Could you check a few things on this model? Use its own coordinates, in mm. A direction names the side the tool comes from. Coordinates: 2 decimals unless noted, no trailing zeros. Write each loop counter-clockwise with the first axis right and the second up, starting at its lowest first coordinate (ties: lowest second). Pieces come first, ordered by that corner, then holes.
Item 1: I want a section at A-A on z = -30. Please give me the cut outline in (x, y), then the cut area to 3 significant figures.
Item 2: I want a section at C-C on y = 13.5. Please give me the cut outline in (x, z), then the cut area to 3 significant figures.
Item 3: Which directions (+Z, -Z, +X, -X, +Y, -Y) give clear straight access to the entire face, cutting with the end or side of a thin tool? Please do faces 1 (the flat face through (16.35, 17, -27)), 2 (the flat face through (-8.146, 22, -12)), 3 (the flat face through (5, 20, -22)).
Item 4: I want a section at D-D on x = 1. Please give me the cut outline in (y, z).
Item 5: I want a section at B-B on x = 13. Please give me the cut outline in (y, z).
Item 6: If I drill on probe 1 along X at (y, z) = (23.5, -2); probe 2 along Z at (x, y) = (5, 21.5); probe 3 along Y at (x, z) = (30, -2.5), over which ranges is the centre line in solid material (lowest first)?
Item 7: For P1, Ø1, axis at y = 17.5, z = -20, coming from the +X side; P2, Ø4, axis at x = 13, y = 26, coming from the -Z side; P3, Ø9.5, axis at x = 14.5, z = -21.5, coming from the +Y side; P4, Ø1, axis at y = 17, z = -27.5, coming from the +X side, each with a flat end and sliding along its axis, tell me the tip position at first contact or that it passes through.
from build123d import *

# Parameters (mm, degrees)
SKETCH3_W           = 50
SKETCH3_H           = 13
BOSS_EXTRUDE1_DEPTH = 32
BOSS_EXTRUDE2_DEPTH = 32
BOSS_EXTRUDE3_DEPTH = 10
SKETCH8_W           = 9.643905297
SKETCH8_H           = 8.359669373
BOSS_EXTRUDE4_DEPTH = 22


with BuildPart() as part:
    # Sketch3 → Boss-Extrude1 (new body)
    with BuildSketch(Plane.XY):
        with Locations((7.209853726, 4.539889959)):
            Rectangle(SKETCH3_W, SKETCH3_H)
    extrude(amount=-BOSS_EXTRUDE1_DEPTH)

    # Sketch4 → Boss-Extrude2 (add)
    with BuildSketch(Plane.XY):
        Polygon((-8.146240977, 11.039889959), (-8.146240977, 33.039889959), (-2.650375504, 33.039889959), (-2.650375504, 11.039889959), (32.209853726, 11.039889959), (32.209853726, -1.960110041), (-17.790146274, -1.960110041), (-17.790146274, 11.039889959), align=None)
    extrude(amount=-BOSS_EXTRUDE2_DEPTH)

    # Sketch5 → Boss-Extrude3 (add)
    with BuildSketch(Plane(origin=(0, 0, -32), x_dir=(-1, 0, 0), z_dir=(0, 0, -1))):
        Polygon((-16.349624496, 11.039889959), (-16.349624496, 23.039889959), (-8.349624496, 23.039889959), (2.650375504, 33.039889959), (2.650375504, 11.039889959), align=None)
    extrude(amount=-BOSS_EXTRUDE3_DEPTH)

    # Sketch8 → Boss-Extrude4 (add)
    with BuildSketch(Plane(origin=(0, 11.039889959, 0), x_dir=(1, 0, 0), z_dir=(0, 1, 0))):
        with Locations((-12.968193625, 27.820165313)):
            Rectangle(SKETCH8_W, SKETCH8_H)
    extrude(amount=BOSS_EXTRUDE4_DEPTH)


solid = part.part
Response values:
1. outline: (-17.79, -1.96) - (32.21, -1.96) - (32.21, 11.04) - (16.35, 11.04) - (16.35, 23.04) - (8.35, 23.04) - (-2.65, 33.04) - (-17.79, 33.04) - close
1. area: 1,270 mm2
2. outline: (-17.79, -32) - (16.35, -32) - (16.35, -22) - (-2.65, -22) - (-2.65, 0) - (-8.15, 0) - (-8.15, -23.64) - (-17.79, -23.64) - close
2. area: 446 mm2
3. face 1: +Z, -Z, +X, +Y
3. face 2: +Z, -X, +Y
3. face 3: +Z, +X, +Y
4. outline: (-1.96, -32) - (29.72, -32) - (29.72, -22) - (11.04, -22) - (11.04, 0) - (-1.96, 0) - close
5. outline: (-1.96, -32) - (23.04, -32) - (23.04, -22) - (11.04, -22) - (11.04, 0) - (-1.96, 0) - close
6. probe 1: x = -8.15 to -2.65
6. probe 2: z = -32 to -22
6. probe 3: y = -1.96 to 11.04
7. P1: stops at x = -2.65
7. P2: passes through
7. P3: stops at y = 23.04
7. P4: stops at x = 16.35
